from build123d import *

# Parameters (mm, degrees)
F0_R      = 69
F1_DEPTH  = 5
F2_R      = 60.5
F3_DEPTH  = 7
F4_R      = 6.25
F5_DEPTH  = 8.5
F6_R      = 3
F7_DEPTH  = 25
F9_DEPTH  = 8.5
F10_R     = 3
F11_DEPTH = 25
F12_SIZE  = 2


with BuildPart() as f1:
    # F0 (on Front) → F1 (new body)
    with BuildSketch(Plane.XZ):
        Circle(F0_R)
    extrude(amount=F1_DEPTH)

    # F2 (on face) → F3 (join)
    with BuildSketch(Plane.XZ.offset(5)):
        Circle(F2_R)
    extrude(amount=F3_DEPTH)

    # F4 (on face) → F5 (cut)
    with BuildSketch(Plane(origin=(0, 0, 0), x_dir=(-1, 0, 0), z_dir=(0, 1, 0))):
        Circle(F4_R)
    extrude(amount=-F5_DEPTH, mode=Mode.SUBTRACT)

    # F6 (on face) → F7 (cut)
    with BuildSketch(Plane.XZ.offset(12)):
        Circle(F6_R)
    extrude(amount=-F7_DEPTH, mode=Mode.SUBTRACT)

    # F8 (on face) → F9 (cut)
    with BuildSketch(Plane(origin=(0, 0, 0), x_dir=(-1, 0, 0), z_dir=(0, 1, 0))):
        with BuildLine():
            ThreePointArc((6.25, -30.5), (4.419417, -26.080583), (0, -24.25))
            Line((0, -24.25), (0, -36.75))
            ThreePointArc((0, -36.75), (4.419417, -34.919417), (6.25, -30.5))
        make_face()
        with BuildLine():
            Line((0, -36.75), (0, -24.25))
            ThreePointArc((0, -24.25), (-6.25, -30.5), (0, -36.75))
        make_face()
    extrude(amount=-F9_DEPTH, mode=Mode.SUBTRACT)

    # F10 (on face) → F11 (cut)
    with BuildSketch(Plane(origin=(0, -8.5, 0), x_dir=(-1, 0, 0), z_dir=(0, 1, 0))):
        with Locations((0, -30.5)):
            Circle(F10_R)
    extrude(amount=-F11_DEPTH, mode=Mode.SUBTRACT)

    # F12
    f12_edges = [f1.edges().sort_by_distance(p)[0] for p in [
        (-60.5, -12, 0),
    ]]
    chamfer(f12_edges, length=F12_SIZE)


solid = f1.part
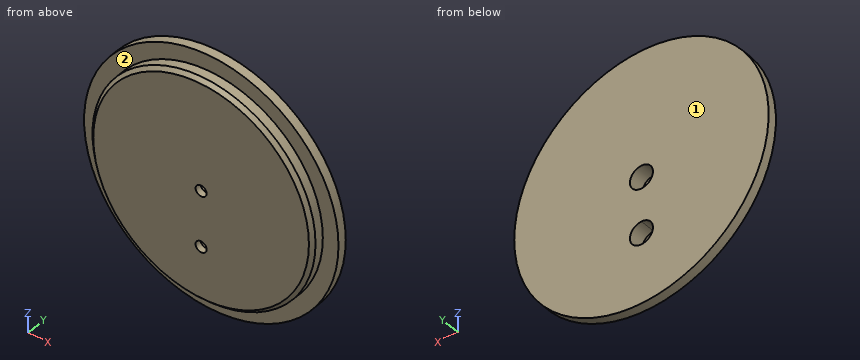
Source: CAD feature listing. Evaluate the final solid. Frame: model axes, mm. Face numbers are marked on the shaded views. A direction names the side the tool comes from. Round coordinates to 2 decimals unless told otherwise and drop trailing zeros. Order: outer loops, then holes, each group sorted by start corner. A loop starts at its lowest first (then second) coordinate and runs counter-clockwise, first axis right, second up. Notation, with made-up numbers: (54, 23) - (85, 23) arc R29 cw to (85, 60) - close; hole circle Ø10 at (-32, 37). An arc over 180 degrees is marked (long way). Use a Markdown table: item, result. Add a question column.
1. Section query B-B (y = -2). Return the cut outline in (x, z), then the cut area to 3 significant figures.
2. First-contact query: pin 1 (1.5 mm diameter, centred on y = -7.5, z = 11, fed in from +X); pin 2 (7 mm diameter, centred on x = 0, z = -30.5, fed in from +Y); pin 3 (2 mm diameter, centred on x = 1, y = -3, fed in from +Z). Flat tips, straight axial feed; report the tip coordinate or a pass-through.
3. Line query: probe 1 along Z at (x, y) = (0, -10); probe 2 along Y at (x, z) = (60, 19); probe 3 along Z at (x, y) = (0, -11.1). Output: solid intervals per line, ascending.
4. Set-up query: the marked faces 1 and 2. Return all of +Z, -Z, +X, -X, +Y, -Y with unobstructed straight access to the full face (end or side cutting, diameter ignored); none if empty.
5. Section query A-A (z = 0). Return the cut outline in (x, y).
Derived:
| question | item | result |
|---|---|---|
| 1 | outline | circle Ø138 at (0, 0); hole (-6.25, -30.5) arc R6.25 ccw to (0, -36.75) arc R6.25 ccw to (0, -24.25) arc R6.25 ccw to start; hole circle Ø12.5 at (0, 0) |
| 1 | area | 14,700 mm2 |
| 2 | pin 1 | x = 59.63 |
| 2 | pin 2 | y = -8.5 |
| 2 | pin 3 | z = 69 |
| 3 | probe 1 | -60.5 to -33.5, -27.5 to -3, 3 to 60.5 |
| 3 | probe 2 | -5 to 0 |
| 3 | probe 3 | -59.4 to -33.5, -27.5 to -3, 3 to 59.4 |
| 4 | face 1 | +Z, -Z, +X, -X, +Y |
| 4 | face 2 | -Y |
| 5 | outline | (-69, -5) - (-60.5, -5) - (-60.5, -10) - (-58.5, -12) - (-3, -12) - (-3, -8.5) - (-6.25, -8.5) - (-6.25, 0) - (-69, 0) - close; (3, -12) - (58.5, -12) - (60.5, -10) - (60.5, -5) - (69, -5) - (69, 0) - (6.25, 0) - (6.25, -8.5) - (3, -8.5) - close |
